from build123d import *

# Parameters (mm, degrees)
SKETCH2_W                                           = 25.4
SKETCH2_H                                           = 63.5
BOSS_EXTRUDE1_DEPTH                                 = 30.17596
SKETCH3_W                                           = 25.4
SKETCH3_H                                           = 21.05
BOSS_EXTRUDE2_DEPTH                                 = 25.4
F_1_4_0_25_DIAMETER_HOLE1_D                         = 6.35
F_1_0MM_DOWEL_HOLE1_D                               = 6.3
F_1_0MM_DOWEL_HOLE1_DEPTH                           = 8.9916
F_1_0MM_DOWEL_HOLE1_TIP                             = 1.89271095
TAP_DRILL_FOR_5_HELICOIL0_D                         = 4
TAP_DRILL_FOR_5_HELICOIL0_DEPTH                     = 15.24
TAP_DRILL_FOR_5_HELICOIL0_TIP                       = 1.201721238
CBORE_FOR_10_BINDING_HEAD_MACHINE_SCREW_D           = 5.1054
CBORE_FOR_10_BINDING_HEAD_MACHINE_SCREW_DEPTH       = 30.17596
CBORE_FOR_10_BINDING_HEAD_MACHINE_SCREW_CBORE_D     = 11.1125
CBORE_FOR_10_BINDING_HEAD_MACHINE_SCREW_CBORE_DEPTH = 5.08


with BuildPart() as part:
    # Sketch2 → Boss-Extrude1 (new body)
    with BuildSketch(Plane(origin=(0, 0, 0), x_dir=(0, 0, -1), z_dir=(1, 0, 0))):
        with Locations((-225.049350785, -379.861725806)):
            Rectangle(SKETCH2_W, SKETCH2_H)
    extrude(amount=-BOSS_EXTRUDE1_DEPTH)

    # Sketch3 → Boss-Extrude2 (add)
    with BuildSketch(Plane.ZY.offset(30.17596)):
        with Locations((225.049350785, -358.636725806)):
            Rectangle(SKETCH3_W, SKETCH3_H)
    extrude(amount=BOSS_EXTRUDE2_DEPTH)

    # 1/4 (0.25) Diameter Hole1 (through all)
    with Locations(Plane(origin=(0, -348.111725806, 0), x_dir=(1, 0, 0), z_dir=(0, 1, 0))):
        with Locations((-42.87596, -225.049350785)):
            Hole(F_1_4_0_25_DIAMETER_HOLE1_D / 2)

    # Ø1.0mm Dowel Hole1
    with Locations(Plane(origin=(0, 0, 0), x_dir=(0, 0, -1), z_dir=(1, 0, 0))):
        with Locations((-231.549350785, -356.861725806), (-218.549350785, -356.861725806), (-218.549350785, -402.861725806), (-231.549350785, -402.861725806)):
            Hole(F_1_0MM_DOWEL_HOLE1_D / 2, depth=F_1_0MM_DOWEL_HOLE1_DEPTH)
            with Locations((0, 0, -(F_1_0MM_DOWEL_HOLE1_DEPTH + F_1_0MM_DOWEL_HOLE1_TIP / 2))):  # 118° drill point
                Cone(0, F_1_0MM_DOWEL_HOLE1_D / 2, F_1_0MM_DOWEL_HOLE1_TIP, mode=Mode.SUBTRACT)

    # Tap Drill for #5 Helicoil0
    with Locations(Plane(origin=(0, 0, 212.349350785), x_dir=(-1, 0, 0), z_dir=(0, 0, -1))):
        with Locations((9.7875, -371.924225806), (9.7875, -387.799225806)):
            Hole(TAP_DRILL_FOR_5_HELICOIL0_D / 2, depth=TAP_DRILL_FOR_5_HELICOIL0_DEPTH)
            with Locations((0, 0, -(TAP_DRILL_FOR_5_HELICOIL0_DEPTH + TAP_DRILL_FOR_5_HELICOIL0_TIP / 2))):  # 118° drill point
                Cone(0, TAP_DRILL_FOR_5_HELICOIL0_D / 2, TAP_DRILL_FOR_5_HELICOIL0_TIP, mode=Mode.SUBTRACT)

    # CBORE for #10 Binding Head Machine Screw1
    with Locations(Plane(origin=(0, 0, 0), x_dir=(0, 0, -1), z_dir=(1, 0, 0))):
        with Locations((-225.049350785, -381.861725806)):
            CounterBoreHole(CBORE_FOR_10_BINDING_HEAD_MACHINE_SCREW_D / 2, CBORE_FOR_10_BINDING_HEAD_MACHINE_SCREW_CBORE_D / 2, CBORE_FOR_10_BINDING_HEAD_MACHINE_SCREW_CBORE_DEPTH, depth=CBORE_FOR_10_BINDING_HEAD_MACHINE_SCREW_DEPTH)


solid = part.part
Can you work these out from the model? Positions are in its coordinate system, mm. A direction names the side the tool comes from. Round coordinates to 2 decimals unless told otherwise and drop trailing zeros. Loops run counter-clockwise (first coordinate to the right, second up) from the corner with the lowest first, then second, coordinate; pieces in that order, holes last. Notation, with made-up numbers: (-20, 8) - (-6, 8) arc R17 cw to (-6, 13) - close; hole circle Ø8 at (-33, 67). An arc over 180 degrees is marked (long way). Answer in a Markdown table with one row per item. Add a question column.
Q1. I want a section at A-A on x = -7. List the corners of the cut face in (y, z) for me, and give its area (3 significant figures).
Q2. For pin 1 Ø3 at (y, z) = (-384, 215) entering from -X; pin 2 Ø1.5 at (x, z) = (-33, 216) entering from -Y; pin 3 Ø2.5 at (x, y) = (-9.79, -387.8) entering from -Z; pin 4 Ø5.5 at (x, z) = (-42.88, 225.05) entering from -Y, each with a flat end and sliding along its axis, tell me the tip position at first contact or that it passes through.
Q3. We'd pull the mould along Z, two halves only. Please class faces 5 (the conical face through (-9.712, -372.263, 228.582)), 6 (the flat face through (-30.176, -390, 225)), 7 (the cylindrical face through (-4.56, -353.74, 231.14)): pulls with the +Z half, pulls with the -Z half, needs draft (parallel to the pull), parting line crosses it, or undercut.
Q4. I want a section at D-D on z = 217.5. Count the separate pieces of the cut face and the enclosed holes in it, and give its area (3 significant figures).
Q5. I want a section at C-C on x = -51. List the corners of the cut face in (y, z) for me.
Q6. I want a section at B-B on z = 214.25. List the corners of the cut face in (x, y) for me, and give its area (3 significant figures).
Q7. I need wall thicknesses on L1, parallel to Z at x = -3, y = -402.5; L2, parallel to X at y = -369.5, z = 230; L3, parallel to Y at x = -43.5, z = 221.25. Which ranges of each line are inside material? Lowest first, please.
Q8. Which directions (+Z, -Z, +X, -X, +Y, -Y) give clear straight access to the entire face, cutting with the end or side of a thin tool? Please do faces 1 (the cylindrical face through (-4.56, -353.74, 218.14)), 2 (the flat face through (-46, -369.162, 228)), 3 (the cylindrical face through (-42.46, -358.78, 221.9)), 4 (the cylindrical face through (-10.22, -389.75, 220.08)).
A:
| question | item | result |
|---|---|---|
| 1 | outline | (-411.61, 212.35) - (-348.11, 212.35) - (-348.11, 237.75) - (-411.61, 237.75) - close; hole circle Ø6.3 at (-402.86, 218.55); hole circle Ø6.3 at (-402.86, 231.55); hole circle Ø5.11 at (-381.86, 225.05); hole circle Ø6.3 at (-356.86, 218.55); hole circle Ø6.3 at (-356.86, 231.55) |
| 1 | area | 1,470 mm^2 |
| 2 | pin 1 | x = -30.18 |
| 2 | pin 2 | y = -369.16 |
| 2 | pin 3 | z = 228.04 |
| 2 | pin 4 | through |
| 3 | face 5 | pulls with the -Z half |
| 3 | face 6 | needs draft |
| 3 | face 7 | undercut |
| 4 | separate pieces | 1 |
| 4 | enclosed holes | 2 |
| 4 | area | 2,310 mm^2 |
| 5 | outline | (-369.16, 212.35) - (-348.11, 212.35) - (-348.11, 237.75) - (-369.16, 237.75) - close |
| 6 | outline | (-55.58, -369.16) - (-30.18, -369.16) - (-30.18, -411.61) - (0, -411.61) - (0, -348.11) - (-55.58, -348.11) - close; hole circle Ø4 at (-9.79, -387.8); hole circle Ø4 at (-9.79, -371.92) |
| 6 | area | 2,430 mm^2 |
| 7 | L1 | 212.35 to 215.42, 221.68 to 228.42, 234.68 to 237.75 |
| 7 | L2 | -30.18 to 0 |
| 7 | L3 | -369.16 to -348.11 |
| 8 | face 1 | +X |
| 8 | face 2 | +Z, -Z, -X, -Y |
| 8 | face 3 | +Y, -Y |
| 8 | face 4 | -Z |
